Design review of the part built by this model. Coordinates are the model's own, in mm. Round coordinates to 2 decimals unless told otherwise and drop trailing zeros. Order: outer loops, then holes, each group sorted by start corner. A loop starts at its lowest first (then second) coordinate and runs counter-clockwise, first axis right, second up. Notation, with made-up numbers: M 78,61 L 126,61 A4 cw 126,67 Z; hole C 40,-35 d5. An arc over 180 degrees is marked long. Use a Markdown table: item, result. Add a question column.
(1) To check wall thickness, follow probe 1 along X at (y, z) = (8, 25); probe 2 along X at (y, z) = (-0.25, 138); probe 3 along Y at (x, z) = (0, 114.5). State the ranges of each line that lie inside material, in increasing order. Write a range as from..to.
(2) For pin 1 (3 mm diameter, centred on x = 1, z = 117, fed in from -Y); pin 2 (1.4 mm diameter, centred on y = -9, z = 73.5, fed in from +X); pin 3 (0.6 mm diameter, centred on x = -17, z = 102.5, fed in from -Y), all flat-tipped, find the tip position at first contact; note any pin that passes through.
(3) Take a section at A-A (x = 0). Write out the cut boundary in (y, z), then the cut area to 3 significant figures.
(4) Take a section at B-B (z = 153). Count the separate pieces of the cut face and the enclosed holes in it, then the cut area to 3 significant figures.
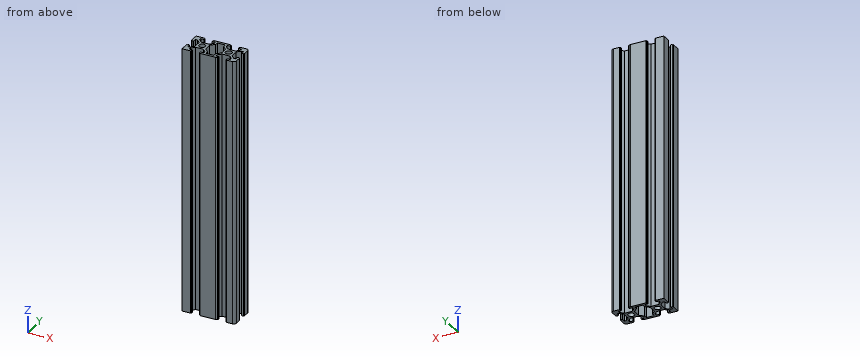
```python
from build123d import *

# Parameters (mm, degrees)
F0_R        = 2.4
F1_DEPTH    = 200
F2_T1_DEPTH = 210
F2_T3_DEPTH = 206.6143782777
F3_R        = 1.5
F4_DEPTH    = 25


# Not quite as in the source:
# - a fillet or chamfer that OpenCascade refuses, or shapes differently, is made with other operations: its cross-section is extruded or revolved along the edge and cut away or added


with BuildPart() as f1:
    # F0 (on Top) → F1 (new body)
    with BuildSketch(Plane.XY):
        Polygon((10, 3.5), (10, 10), (3.5, 10), (3.5, 9.5), (3, 9.5), (3, 8.2), (5.5, 8.2), (5.5, 6.5606601718), (2.9393398282, 4), (0, 4), (-2.9393398282, 4), (-5.5, 6.5606601718), (-5.5, 8.2), (-3, 8.2), (-3, 9.5), (-3.5, 9.5), (-3.5, 10), (-10, 10), (-16.5, 10), (-16.5, 9.5), (-17, 9.5), (-17, 8.2), (-14.5, 8.2), (-14.5, 6.5606601718), (-17.0606601718, 4), (-20, 4), (-22.9393398282, 4), (-25.5, 6.5606601718), (-25.5, 8.2), (-23, 8.2), (-23, 9.5), (-23.5, 9.5), (-23.5, 10), (-30, 10), (-30, 3.5), (-29.5, 3.5), (-29.5, 3), (-28.2, 3), (-28.2, 5.5), (-26.5606601718, 5.5), (-24, 2.9393398282), (-24, -2.9393398282), (-26.5606601718, -5.5), (-28.2, -5.5), (-28.2, -3), (-29.5, -3), (-29.5, -3.5), (-30, -3.5), (-30, -10), (-23.5, -10), (-23.5, -9.5), (-23, -9.5), (-23, -8.2), (-25.5, -8.2), (-25.5, -6.5606601718), (-22.9393398282, -4), (-20, -4), (-17.0606601718, -4), (-14.5, -6.5606601718), (-14.5, -8.2), (-17, -8.2), (-17, -9.5), (-16.5, -9.5), (-16.5, -10), (-10, -10), (-3.5, -10), (-3.5, -9.5), (-3, -9.5), (-3, -8.2), (-5.5, -8.2), (-5.5, -6.5606601718), (-2.9393398282, -4), (0, -4), (2.9393398282, -4), (5.5, -6.5606601718), (5.5, -8.2), (3, -8.2), (3, -9.5), (3.5, -9.5), (3.5, -10), (10, -10), (10, -3.5), (9.5, -3.5), (9.5, -3), (8.2, -3), (8.2, -5.5), (6.5606601718, -5.5), (4, -2.9393398282), (4, 2.9393398282), (6.5606601718, 5.5), (8.2, 5.5), (8.2, 3), (9.5, 3), (9.5, 3.5), align=None)
        with Locations((-20, 0)):
            Circle(F0_R, mode=Mode.SUBTRACT)
        Polygon((-7, 5.9393398282), (-4, 2.9393398282), (-4, -2.797918472), (-7, -5.797918472), (-7, -8.2), (-13, -8.2), (-13, -5.797918472), (-16, -2.797918472), (-16, 2.9393398282), (-13, 5.9393398282), (-13, 8.2), (-7, 8.2), align=None, mode=Mode.SUBTRACT)
        Circle(F0_R, mode=Mode.SUBTRACT)
    extrude(amount=F1_DEPTH)

    # F2: fillet of radius 2 on 4 edges, made by hand

    # F2_s2 → F2_t1 (cut)
    with BuildSketch(Plane.XY.offset(-5)):
        with BuildLine():
            ThreePointArc((8, 10), (9.4142135624, 9.4142135624), (10, 8))
            Line((10, 8), (10, 10))
            Line((10, 10), (8, 10))
        make_face()
        with BuildLine():
            ThreePointArc((10, -8), (9.4142135624, -9.4142135624), (8, -10))
            Line((8, -10), (10, -10))
            Line((10, -10), (10, -8))
        make_face()
    extrude(amount=F2_T1_DEPTH, mode=Mode.SUBTRACT)

    # F2_s4 → F2_t3 (cut)
    with BuildSketch(Plane.XY.offset(-3.3071891388)):
        with BuildLine():
            ThreePointArc((-3.5, -9.5), (-4.1157688743, -9.8708286934), (-4.8228756555, -10))
            Line((-4.8228756555, -10), (-3.5, -10))
            Line((-3.5, -10), (-3.5, -9.5))
        make_face()
        with BuildLine():
            ThreePointArc((-4.8228756555, 10), (-4.1157688743, 9.8708286934), (-3.5, 9.5))
            Line((-3.5, 9.5), (-3.5, 10))
            Line((-3.5, 10), (-4.8228756555, 10))
        make_face()
    extrude(amount=F2_T3_DEPTH, mode=Mode.SUBTRACT)

    # F3 (on face) → F4 (cut)
    with BuildSketch(Plane.YZ.offset(4)):
        with Locations((0, 190.370157361)):
            Circle(F3_R)
    extrude(amount=-F4_DEPTH, mode=Mode.SUBTRACT)


solid = f1.part
```
Verdict:
| question | item | result |
|---|---|---|
| 1 | probe 1 | x = -30..-25.5, -14.5..-13, -7..-5.5, 5.5..10 |
| 1 | probe 2 | x = -24..-22.39, -17.61..-16, -4..-2.39, 2.39..4 |
| 1 | probe 3 | y = -4..-2.4, 2.4..4 |
| 2 | pin 1 | stops at y = -4 |
| 2 | pin 2 | stops at x = 9.98 |
| 2 | pin 3 | stops at y = -9.5 |
| 3 | outline | M -4,0 L -2.4,0 L -2.4,200 L -4,200 Z; M 2.4,0 L 4,0 L 4,200 L 2.4,200 Z |
| 3 | area | 640 mm^2 |
| 4 | separate pieces | 1 |
| 4 | enclosed holes | 3 |
| 4 | area | 305 mm^2 |
